```python
from build123d import *

# Parameters (mm, degrees)
F0_W        = 76.2
F0_H        = 19.05
F1_DEPTH    = 19.05
F3_D        = 12.7
F3_DEPTH    = 39.1412730195
F5_D        = 12.7
F6_T1_DEPTH = 101.6


# Not quite as in the source:
# - a fillet or chamfer that OpenCascade refuses, or shapes differently, is made with other operations: its cross-section is extruded or revolved along the edge and cut away or added


with BuildPart() as f1:
    # F0 (on Top) → F1 (new body)
    with BuildSketch(Plane.XY):
        with Locations((1.0402730195, 0)):
            Rectangle(F0_W, F0_H)
    extrude(amount=F1_DEPTH)

    # F3 (through all, one way)
    with BuildSketch(Plane(origin=(0, 0, 0), x_dir=(0, 1, 0), z_dir=(-1, 0, 0))):
        with Locations((0, -9.525)):
            Circle(F3_D / 2)
    extrude(amount=-F3_DEPTH, mode=Mode.SUBTRACT)

    # F5 (through all)
    with Locations(Plane(origin=(0, 0, 0), x_dir=(1, 0, 0), z_dir=(0, 0, -1))):
        with Locations((-27.5347269805, 0)):
            Hole(F5_D / 2)

    # F6: fillet of radius 5.08 on 4 edges, made by hand

    # F6_s2 → F6_t1 (cut)
    with BuildSketch(Plane.YZ.offset(-49.7597269805)):
        with BuildLine():
            ThreePointArc((4.445, 19.05), (8.0371024484, 17.5621024484), (9.525, 13.97))
            Line((9.525, 13.97), (9.525, 19.05))
            Line((9.525, 19.05), (4.445, 19.05))
        make_face()
        with BuildLine():
            ThreePointArc((-9.525, 13.97), (-8.0371024484, 17.5621024484), (-4.445, 19.05))
            Line((-4.445, 19.05), (-9.525, 19.05))
            Line((-9.525, 19.05), (-9.525, 13.97))
        make_face()
        with BuildLine():
            ThreePointArc((-9.525, 5.08), (-8.0371024484, 1.4878975516), (-4.445, 0))
            Line((-4.445, 0), (-9.525, 0))
            Line((-9.525, 0), (-9.525, 5.08))
        make_face()
        with BuildLine():
            ThreePointArc((4.445, 0), (8.0371024484, 1.4878975516), (9.525, 5.08))
            Line((9.525, 5.08), (9.525, 0))
            Line((9.525, 0), (4.445, 0))
        make_face()
    extrude(amount=F6_T1_DEPTH, mode=Mode.SUBTRACT)


solid = f1.part
```
Could you check a few things on this model? Use its own coordinates, in mm. A direction names the side the tool comes from. Give positions to 0.01 mm unless a question says otherwise; leave off trailing zeros. Loops run counter-clockwise (first coordinate to the right, second up) from the corner with the lowest first, then second, coordinate; pieces in that order, holes last. Notation, with made-up numbers: (-34, 87.5) -> (24, 87.5) arc R19 cw to (24, 112.5) -> close; hole circle Ø4 at (25.25, 72.5). An arc over 180 degrees is marked (long way). Put each result on its own line as item: value.
(1) Imagine slicing it at A-A on y = 0. Write out the boundary of the cut face in (x, z) (3 decimals), plus the area to 3 significant figures.
Computed:
outline: (-37.06, 0) -> (-33.885, 0) -> (-33.885, 19.05) -> (-37.06, 19.05) -> close; (-21.185, 0) -> (39.14, 0) -> (39.14, 3.175) -> (0, 3.175) -> (0, 15.875) -> (39.14, 15.875) -> (39.14, 19.05) -> (-21.185, 19.05) -> close
area: 713 mm^2
(2) I'm going to push a flat-ended pin straight in: pin 1 Ø2 at (x, y) = (12, -7) entering from +Z. Where does the tip first touch, or does it pass through?
Computed:
pin 1: z = 18.81
(3) Imagine slicing it at C-C on x = -7.5. Write out the boundary of the cut face in (y, z) (3 decimals), plus the area to 3 significant figures.
Computed:
outline: (-9.525, 5.08) arc R5.08 ccw to (-4.445, 0) -> (4.445, 0) arc R5.08 ccw to (9.525, 5.08) -> (9.525, 13.97) arc R5.08 ccw to (4.445, 19.05) -> (-4.445, 19.05) arc R5.08 ccw to (-9.525, 13.97) -> close
area: 341 mm^2
(4) Imagine slicing it at D-D on y = 3.25. Write out the boundary of the cut face in (x, z), plus the area to 3 significant figures.
Computed:
outline: (-37.06, 0) -> (-32.99, 0) -> (-32.99, 19.05) -> (-37.06, 19.05) -> close; (-22.08, 0) -> (39.14, 0) -> (39.14, 4.07) -> (0, 4.07) -> (0, 14.98) -> (39.14, 14.98) -> (39.14, 19.05) -> (-22.08, 19.05) -> close
area: 817 mm^2
(5) Thinking about a two-plate mould opening in Z: for faces 3 (the face through (-33.59, -1.91, 9.66)), 4 (the face through (19.3, -0.83, 3.23)), 5 (the face through (8, 0, 0)), 6 (the face through (-35, 0, 19.05)), which applies, pulls with the +Z half, pulls with the -Z half, needs draft (parallel to the pull), parting line crosses it, or undercut?
Computed:
face 3: needs draft
face 4: undercut
face 5: pulls with the -Z half
face 6: pulls with the +Z half
(6) For faces 1 (the face through (0.51, -8.08, 1.53)), 2 (the face through (0, 0, 9)), which set-ups out of +Z, -Z, +X, -X, +Y, -Y let a thin tool reach every point of the face, with its end or its side?
Computed:
face 1: -Z, +X, -X, -Y
face 2: +X
(7) Imagine slicing it at B-B on x = 24.5. Write out the boundary of the cut face in (y, z) (3 decimals).
Computed:
outline: (-9.525, 5.08) arc R5.08 ccw to (-4.445, 0) -> (4.445, 0) arc R5.08 ccw to (9.525, 5.08) -> (9.525, 13.97) arc R5.08 ccw to (4.445, 19.05) -> (-4.445, 19.05) arc R5.08 ccw to (-9.525, 13.97) -> close; hole circle Ø12.7 at (0, 9.525)
(8) Please list where these lines run through material, in increasing order: probe 1 along Z at (x, y) = (11.5, 0) (3 decimals); probe 2 along X at (y, z) = (0.25, 1.25); probe 3 along Z at (x, y) = (-4.5, 4.75). Write a range as [from, to].
Computed:
probe 1: [0, 3.175], [15.875, 19.05]
probe 2: [-37.06, -33.88], [-21.19, 39.14]
probe 3: [0.01, 19.04]
